```python
from build123d import *

# Parameters (mm, degrees)
Y_KSEKLIK_EKSTR_ZYON1_DEPTH = 5


with BuildPart() as part:
    # Çizim1 → Yükseklik-Ekstrüzyon1 (new body)
    with BuildSketch(Plane.XY.offset(4.115610561)):
        Polygon((-4.7, 0.140638796), (-4.7, -6.859361204), (4.7, -6.859361204), (4.7, 0.140638796), (2.309401077, -4), (-2.309401077, -4), align=None)
    extrude(amount=Y_KSEKLIK_EKSTR_ZYON1_DEPTH)


solid = part.part
```
The model under review builds one solid part; all positions refer to its coordinate system, in mm. A direction names the side the tool comes from. Round coordinates to 2 decimals unless told otherwise and drop trailing zeros. Order: outer loops, then holes, each group sorted by start corner. A loop starts at its lowest first (then second) coordinate and runs counter-clockwise, first axis right, second up. Notation, with made-up numbers: (86.25, -31.75) -> (99.25, -31.75) arc R14 cw to (99.25, -11.75) -> close; hole circle Ø8 at (87.5, 37.25). An arc over 180 degrees is marked (long way). One line per item, written item: value. Start each with the question number.
Q1. Take a section at B-B (z = 7.85). Write out the cut boundary in (x, y), and give its area (3 significant figures).
Q2. Take a section at A-A (y = -1). Write out the cut boundary in (x, z).
Q3. Wall thickness on line 1 (X direction, y = -1, z = 7.3); line 2 (Y direction, x = -1, z = 7.9); line 3 (X direction, y = -2, z = 6.8): over which ranges is each line inside the solid? List them lowest first.
Q4. Clearance check with a flat-ended pin moving along its axis: pin 1 Ø1.5 at (x, y) = (1, -2) entering from -Z. State where the tip first meets the part, or that it passes through.
Q5. Machinability: for faces 1 (the face through (-3.488, -1.959, 6.581)), 2 (the face through (0, -5, 9.116)), which of the approach directions +Z, -Z, +X, -X, +Y, -Y give a long, thin tool a straight path to every point of the face, cutting with its end or side? Answer none if there is none.
Q6. Take a section at C-C (x = -0.5). Write out the cut boundary in (y, z), and give its area (3 significant figures).
Q7. Take a section at D-D (y = -0.25). Write out the cut boundary in (x, z).
Q8. Mouldability with a two-part tool opening along X and no side actions: class faces 3 (the face through (3.52, -1.9, 6.58)), 4 (the face through (-4.7, -3, 7)), 5 (the face through (0, -6.859, 7)) as released by +X, released by -X, zero draft, split by the parting line, or undercut.
Reported:
1. outline: (-4.7, -6.86) -> (4.7, -6.86) -> (4.7, 0.14) -> (2.31, -4) -> (-2.31, -4) -> (-4.7, 0.14) -> close
1. area: 36.8 mm2
2. outline: (-4.7, 4.12) -> (-4.04, 4.12) -> (-4.04, 9.12) -> (-4.7, 9.12) -> close; (4.04, 4.12) -> (4.7, 4.12) -> (4.7, 9.12) -> (4.04, 9.12) -> close
3. line 1: x = -4.7 to -4.04, 4.04 to 4.7
3. line 2: y = -6.86 to -4
3. line 3: x = -4.7 to -3.46, 3.46 to 4.7
4. pin 1: passes through
5. face 1: +Z, -Z, +Y
5. face 2: +Z, +X, -X, +Y, -Y
6. outline: (-6.86, 4.12) -> (-4, 4.12) -> (-4, 9.12) -> (-6.86, 9.12) -> close
6. area: 14.3 mm2
7. outline: (-4.7, 4.12) -> (-4.47, 4.12) -> (-4.47, 9.12) -> (-4.7, 9.12) -> close; (4.47, 4.12) -> (4.7, 4.12) -> (4.7, 9.12) -> (4.47, 9.12) -> close
8. face 3: undercut
8. face 4: released by -X
8. face 5: zero draft
